Source: CAD feature listing. Evaluate the final solid. Frame: model axes, mm. A direction names the side the tool comes from. Give positions to 0.01 mm unless a question says otherwise; leave off trailing zeros. Order: outer loops, then holes, each group sorted by start corner. A loop starts at its lowest first (then second) coordinate and runs counter-clockwise, first axis right, second up. Notation, with made-up numbers: (-33, 0) -> (0, 0) arc R20 cw to (0, 37) -> close; hole circle Ø9 at (63.25, 40.5). An arc over 180 degrees is marked (long way). Use CSV: the item, a comma, the result in double quotes.
```python
from build123d import *

# Parameters (mm, degrees)
SKETCH_1_W          = 35
SKETCH_1_H          = 10
SKETCH_1_R          = 1.5
EXTRUDE_1_DEPTH     = 8
CUT_EXTRUDE_START   = -1.5
SKETCH_2_R          = 3
SKETCH_2_R_2        = 1.5
CUT_EXTRUDE_1_DEPTH = 1.5
SKETCH_3_W          = 35
SKETCH_3_H          = 6
EXTRUDE_2_DEPTH     = 8
CUT_EXTRUDE_2_DEPTH = 38.549966711
FILLET_2_R          = 3


with BuildPart() as part:
    # 草图1 → 凸台-拉伸1 (new body)
    with BuildSketch(Plane.XY):
        Rectangle(SKETCH_1_W, SKETCH_1_H)
        with Locations((-5, 0)):
            Circle(SKETCH_1_R, mode=Mode.SUBTRACT)
        with Locations(Location((5, 0, 0), (0, 0, 180))):
            Circle(SKETCH_1_R, mode=Mode.SUBTRACT)
    extrude(amount=EXTRUDE_1_DEPTH)

    # 草图2 → 切除-拉伸1 (cut)
    # profile 1 of 2: a face of its own
    with BuildSketch(Plane.XY.offset(8).offset(CUT_EXTRUDE_START)):
        with Locations((-5, 0)):
            Circle(SKETCH_2_R)
        with Locations((-5, 0)):
            Circle(SKETCH_2_R_2, mode=Mode.SUBTRACT)
    # profile 2 of 2: a face of its own
    with BuildSketch(Plane.XY.offset(8).offset(CUT_EXTRUDE_START)):
        with Locations((5, 0)):
            Circle(SKETCH_2_R)
        with Locations(Location((5, 0, 0), (0, 0, 180))):
            Circle(SKETCH_2_R_2, mode=Mode.SUBTRACT)
    extrude(amount=CUT_EXTRUDE_1_DEPTH, mode=Mode.SUBTRACT)

    # 草图3 → 凸台-拉伸2 (add)
    with BuildSketch(Plane.XY.offset(8)):
        with Locations((0, -8)):
            Rectangle(SKETCH_3_W, SKETCH_3_H)
    extrude(amount=-EXTRUDE_2_DEPTH)

    # 草图4 → 切除-拉伸2 (cut, through all)
    with BuildSketch(Plane.ZY.offset(17.5)):
        Polygon((8, 5), (7.5, 5), (8, -11), align=None)
    extrude(amount=-CUT_EXTRUDE_2_DEPTH, mode=Mode.SUBTRACT)

    # 圆角2
    fillet_2_edges = [part.edges().sort_by_distance(p)[0] for p in [
        (0, -11, 8),
        (-17.5, -11, 4),
        (17.5, -11, 4),
        (-17.5, 5, 3.75),
        (17.5, 5, 3.75),
    ]]
    fillet(fillet_2_edges, radius=FILLET_2_R)


solid = part.part
```
1. Mould query, pull axis X, two halves, no side actions, for faces 1 (the cylindrical face through (16.6, -10.14, 3.02)), 2 (the cylindrical face through (-3.616, -2.662, 7.126)), 3 (the flat face through (-17.5, -3, 4)). Classes: released by +X, released by -X, zero draft, split by the parting line, or undercut.
Answer below:
face 1,"released by +X"
face 2,"undercut"
face 3,"released by -X"
2. Access query for faces 4 (the flat face through (6.3, -1.3, 6.5)), 5 (the flat face through (17.5, -3, 4)). Directions: +Z, -Z, +X, -X, +Y, -Y. A direction counts if a zero-diameter tool reaches every point of the face in a straight line with its end or side. Return the directions, or none.
Answer below:
face 4,"+Z"
face 5,"+Z, -Z, +X, +Y, -Y"
3. Ray query, line 1 along X through (y, z) = (0, 7.2); line 2 along Z through (x, y) = (-14, -9.5); line 3 along Y through (x, z) = (-5, 4.5). Return the intervals inside material, ascending.
Answer below:
line 1,"x = -17.5 to -8, -2 to 2, 8 to 17.5"
line 2,"z = 0 to 7.5"
line 3,"y = -11 to -1.5, 1.5 to 5"
4. Section query C-C on x = 13.5. Return loops of the section in (y, z), plus the area to 3 significant figures.
Answer below:
outline,"(-11, 0) -> (5, 0) -> (5, 7.5) -> (-7.91, 7.9) arc R3 ccw to (-11, 4.9) -> close"
area,"122 mm²"
5. Pin query (flat end, axial travel): P1, Ø5, axis at x = 2, y = 0, coming from the +Z side; P2, Ø1.8, axis at x = -4, y = 1, coming from the +Z side; P3, Ø6.5, axis at x = 4, y = -1, coming from the +Z side. Return the tip coordinate at first contact, or that it passes through.
Answer below:
P1,"stops at z = 7.73"
P2,"stops at z = 6.5"
P3,"stops at z = 7.79"
6. Section query B-B on x = 5. Return loops of the section in (y, z).
Answer below:
outline,"(-11, 0) -> (-1.5, 0) -> (-1.5, 6.5) -> (-3, 6.5) -> (-3, 7.75) -> (-7.91, 7.9) arc R3 ccw to (-11, 4.9) -> close; (1.5, 0) -> (5, 0) -> (5, 7.5) -> (3, 7.56) -> (3, 6.5) -> (1.5, 6.5) -> close"
7. Section query D-D on z = 5.25. Return loops of the section in (x, y), plus the area to 3 significant figures.
Answer below:
outline,"(-17.5, -8) arc R3 ccw to (-14.85, -10.98) -> (14.85, -10.98) arc R3 ccw to (17.5, -8) -> (17.5, 2) arc R3 ccw to (14.5, 5) -> (-14.5, 5) arc R3 ccw to (-17.5, 2) -> close; hole circle Ø3 at (-5, 0); hole circle Ø3 at (5, 0)"
area,"538 mm²"
8. Section query A-A on z = 2. Return loops of the section in (x, y).
Answer below:
outline,"(-17.5, -8) arc R3 ccw to (-14.5, -11) -> (14.5, -11) arc R3 ccw to (17.5, -8) -> (17.5, 2) arc R3 ccw to (14.5, 5) -> (-14.5, 5) arc R3 ccw to (-17.5, 2) -> close; hole circle Ø3 at (-5, 0); hole circle Ø3 at (5, 0)"
